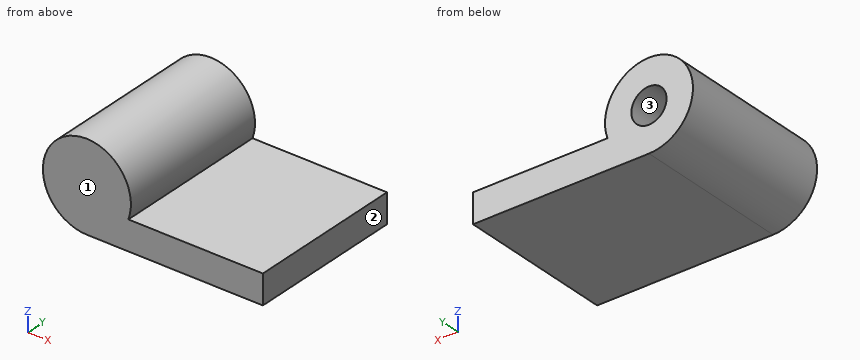
from build123d import *

# Parameters (mm, degrees)
SKETCH_1_R      = 3
EXTRUDE_1_DEPTH = 10.8
SKETCH_7_W      = 2
SKETCH_7_H      = 10.8
EXTRUDE_2_DEPTH = 12
ST2_2_1_D       = 2.4
ST2_2_1_DEPTH   = 8
ST2_2_1_TIP     = 0.721032743


with BuildPart() as part:
    # 草图1 → 凸台-拉伸1 (new body)
    with BuildSketch(Plane(origin=(0, 0, 0), x_dir=(1, 0, 0), z_dir=(0, 1, 0))):
        with Locations(Location((0, 0, 0), (0, 0, 90))):
            Circle(SKETCH_1_R)
    extrude(amount=EXTRUDE_1_DEPTH)

    # 草图7 → 凸台-拉伸2 (add)
    with BuildSketch(Plane(origin=(0, 0, 0), x_dir=(0, 0, -1), z_dir=(1, 0, 0))):
        with Locations((2, 5.4)):
            Rectangle(SKETCH_7_W, SKETCH_7_H)
    extrude(amount=EXTRUDE_2_DEPTH)

    # ST2.2 间隙孔1
    with Locations(Plane.ZX.offset(10.8)):
        with Locations((0, 0)):
            Hole(ST2_2_1_D / 2, depth=ST2_2_1_DEPTH)
            with Locations((0, 0, -(ST2_2_1_DEPTH + ST2_2_1_TIP / 2))):  # 118° drill point
                Cone(0, ST2_2_1_D / 2, ST2_2_1_TIP, mode=Mode.SUBTRACT)


solid = part.part
Can you work these out from the model? Positions are in its coordinate system, mm. Face numbers are marked on the shaded views. Coordinates: 2 decimals unless noted, no trailing zeros. Write each loop counter-clockwise with the first axis right and the second up, starting at its lowest first coordinate (ties: lowest second). Pieces come first, ordered by that corner, then holes. Notation, with made-up numbers: (-38.75, 27.25) - (9.25, 27.25) arc R28 ccw to (9.25, 58.25) - close; hole circle Ø4 at (-15, 85). An arc over 180 degrees is marked (long way). Return JSON: item names as keys, results as strings. Group by question number.
Item 1: If we section it at C-C (z = 1.65): Write out the boundary of the cut face in (x, y), then the cut area to 3 significant figures.
Item 2: If we section it at A-A (y = 10.25): Write out the boundary of the cut face in (x, z), then the cut area to 3 significant figures.
Item 3: I'm going to push flat-ended pins straight in: pin 1 Ø1.5 at (x, y) = (9.5, 9) entering from +Z; pin 2 Ø1 at (x, z) = (3, -2.5) entering from -Y. Where does each tip first touch, or does it pass through?
Item 4: We'd pull the mould along X, two halves only. Please class the marked faces 1, 2 and 3: pulls with the +X half, pulls with the -X half, needs draft (parallel to the pull), parting line crosses it, or undercut.
Item 5: If we section it at B-B (x = 8.25): Write out the boundary of the cut face in (y, z), then the cut area to 3 significant figures.
Item 6: Please list where these lines run through material, in increasing order: probe 1 along X at (y, z) = (6.5, 0); probe 2 along Z at (x, y) = (9.5, 8); probe 3 along Z at (x, y) = (-0.5, 8.25).
Return value:
{
 "1": {"outline": "(-2.51, 0) - (2.51, 0) - (2.51, 10.8) - (-2.51, 10.8) - close", "area": "54.1 mm^2"},
 "2": {"outline": "(0, -3) - (12, -3) - (12, -1) - (2.83, -1) arc R3 ccw (long way) to start; hole circle Ø2.4 at (0, 0)", "area": "43.6 mm^2"},
 "3": {"pin 1": "stops at z = -1", "pin 2": "stops at y = 0"},
 "4": {"face 1": "needs draft", "face 2": "pulls with the +X half", "face 3": "undercut"},
 "5": {"outline": "(0, -3) - (10.8, -3) - (10.8, -1) - (0, -1) - close", "area": "21.6 mm^2"},
 "6": {"probe 1": "x = -3 to -1.2, 1.2 to 3", "probe 2": "z = -3 to -1", "probe 3": "z = -2.96 to -1.09, 1.09 to 2.96"}
}
